```python
from build123d import *

# Parameters (mm, degrees)
EXTRUDE_2_DEPTH     = 3
SKETCH_1_R          = 3.5
CUT_EXTRUDE_2_DEPTH = 4
SKETCH_2_R          = 6.5
CUT_EXTRUDE_4_DEPTH = 2


with BuildPart() as part:
    # Эскиз3 → Бобышка-Вытянуть2 (new body)
    with BuildSketch(Plane(origin=(0, 0, 0), x_dir=(1, 0, 0), z_dir=(0, 1, 0))):
        with BuildLine():
            ThreePointArc((-6.4739783, 66.952525078), (0, 69.5), (6.4739783, 66.952525078))
            ThreePointArc((6.4739783, 66.952525078), (8.677759132, 65.914124613), (11.075205769, 66.34676199))
            ThreePointArc((11.075205769, 66.34676199), (17.987923635, 67.131844927), (23.581971447, 62.995584227))
            ThreePointArc((23.581971447, 62.995584227), (25.441902451, 61.422185949), (27.869632868, 61.219576716))
            ThreePointArc((27.869632868, 61.219576716), (34.75, 60.188765563), (39.082892211, 54.745598415))
            ThreePointArc((39.082892211, 54.745598415), (40.472222163, 52.744426818), (42.764790543, 51.920378458))
            ThreePointArc((42.764790543, 51.920378458), (49.143921292, 49.143921292), (51.920378458, 42.764790543))
            ThreePointArc((51.920378458, 42.764790543), (52.744426818, 40.472222163), (54.745598415, 39.082892211))
            ThreePointArc((54.745598415, 39.082892211), (60.188765563, 34.75), (61.219576716, 27.869632868))
            ThreePointArc((61.219576716, 27.869632868), (61.422185949, 25.441902451), (62.995584227, 23.581971447))
            ThreePointArc((62.995584227, 23.581971447), (67.131844927, 17.987923635), (66.34676199, 11.075205769))
            ThreePointArc((66.34676199, 11.075205769), (65.914124613, 8.677759132), (66.952525078, 6.4739783))
            ThreePointArc((66.952525078, 6.4739783), (69.5, 0), (66.952525078, -6.4739783))
            ThreePointArc((66.952525078, -6.4739783), (65.914124613, -8.677759132), (66.34676199, -11.075205769))
            ThreePointArc((66.34676199, -11.075205769), (67.131844927, -17.987923635), (62.995584227, -23.581971447))
            ThreePointArc((62.995584227, -23.581971447), (61.422185949, -25.441902451), (61.219576716, -27.869632868))
            ThreePointArc((61.219576716, -27.869632868), (60.188765563, -34.75), (54.745598415, -39.082892211))
            ThreePointArc((54.745598415, -39.082892211), (52.744426818, -40.472222163), (51.920378458, -42.764790543))
            ThreePointArc((51.920378458, -42.764790543), (49.143921292, -49.143921292), (42.764790543, -51.920378458))
            ThreePointArc((42.764790543, -51.920378458), (40.472222163, -52.744426818), (39.082892211, -54.745598415))
            ThreePointArc((39.082892211, -54.745598415), (34.75, -60.188765563), (27.869632868, -61.219576716))
            ThreePointArc((27.869632868, -61.219576716), (25.441902451, -61.422185949), (23.581971447, -62.995584227))
            ThreePointArc((23.581971447, -62.995584227), (17.987923635, -67.131844927), (11.075205769, -66.34676199))
            ThreePointArc((11.075205769, -66.34676199), (8.677759132, -65.914124613), (6.4739783, -66.952525078))
            ThreePointArc((6.4739783, -66.952525078), (0, -69.5), (-6.4739783, -66.952525078))
            ThreePointArc((-6.4739783, -66.952525078), (-8.677759132, -65.914124613), (-11.075205769, -66.34676199))
            ThreePointArc((-11.075205769, -66.34676199), (-17.987923635, -67.131844927), (-23.581971447, -62.995584227))
            ThreePointArc((-23.581971447, -62.995584227), (-25.441902451, -61.422185949), (-27.869632868, -61.219576716))
            ThreePointArc((-27.869632868, -61.219576716), (-34.75, -60.188765563), (-39.082892211, -54.745598415))
            ThreePointArc((-39.082892211, -54.745598415), (-40.472222163, -52.744426818), (-42.764790543, -51.920378458))
            ThreePointArc((-42.764790543, -51.920378458), (-49.143921292, -49.143921292), (-51.920378458, -42.764790543))
            ThreePointArc((-51.920378458, -42.764790543), (-52.744426818, -40.472222163), (-54.745598415, -39.082892211))
            ThreePointArc((-54.745598415, -39.082892211), (-60.188765563, -34.75), (-61.219576716, -27.869632868))
            ThreePointArc((-61.219576716, -27.869632868), (-61.422185949, -25.441902451), (-62.995584227, -23.581971447))
            ThreePointArc((-62.995584227, -23.581971447), (-67.131844927, -17.987923635), (-66.34676199, -11.075205769))
            ThreePointArc((-66.34676199, -11.075205769), (-65.914124613, -8.677759132), (-66.952525078, -6.4739783))
            ThreePointArc((-66.952525078, -6.4739783), (-69.5, 0), (-66.952525078, 6.4739783))
            ThreePointArc((-66.952525078, 6.4739783), (-65.914124613, 8.677759132), (-66.34676199, 11.075205769))
            ThreePointArc((-66.34676199, 11.075205769), (-67.131844927, 17.987923635), (-62.995584227, 23.581971447))
            ThreePointArc((-62.995584227, 23.581971447), (-61.422185949, 25.441902451), (-61.219576716, 27.869632868))
            ThreePointArc((-61.219576716, 27.869632868), (-60.188765563, 34.75), (-54.745598415, 39.082892211))
            ThreePointArc((-54.745598415, 39.082892211), (-52.744426818, 40.472222163), (-51.920378458, 42.764790543))
            ThreePointArc((-51.920378458, 42.764790543), (-49.143921292, 49.143921292), (-42.764790543, 51.920378458))
            ThreePointArc((-42.764790543, 51.920378458), (-40.472222163, 52.744426818), (-39.082892211, 54.745598415))
            ThreePointArc((-39.082892211, 54.745598415), (-34.75, 60.188765563), (-27.869632868, 61.219576716))
            ThreePointArc((-27.869632868, 61.219576716), (-25.441902451, 61.422185949), (-23.581971447, 62.995584227))
            ThreePointArc((-23.581971447, 62.995584227), (-17.987923635, 67.131844927), (-11.075205769, 66.34676199))
            ThreePointArc((-11.075205769, 66.34676199), (-8.677759132, 65.914124613), (-6.4739783, 66.952525078))
        make_face()
    extrude(amount=EXTRUDE_2_DEPTH)

    # Эскиз1 → Вырез-Вытянуть2 (cut, through all)
    with BuildSketch(Plane(origin=(0, 0, 0), x_dir=(1, 0, 0), z_dir=(0, 1, 0))):
        with Locations((0, 60)):
            Circle(SKETCH_1_R)
        with Locations((15.529142706, 57.955549577)):
            Circle(SKETCH_1_R)
        with Locations((30, 51.961524227)):
            Circle(SKETCH_1_R)
        with Locations((42.426406871, 42.426406871)):
            Circle(SKETCH_1_R)
        with Locations((51.961524227, 30)):
            Circle(SKETCH_1_R)
        with Locations((57.955549577, 15.529142706)):
            Circle(SKETCH_1_R)
        with Locations((60, 0)):
            Circle(SKETCH_1_R)
        with Locations((57.955549577, -15.529142706)):
            Circle(SKETCH_1_R)
        with Locations((51.961524227, -30)):
            Circle(SKETCH_1_R)
        with Locations((42.426406871, -42.426406871)):
            Circle(SKETCH_1_R)
        with Locations((30, -51.961524227)):
            Circle(SKETCH_1_R)
        with Locations((15.529142706, -57.955549577)):
            Circle(SKETCH_1_R)
        with Locations((0, -60)):
            Circle(SKETCH_1_R)
        with Locations((-15.529142706, -57.955549577)):
            Circle(SKETCH_1_R)
        with Locations((-30, -51.961524227)):
            Circle(SKETCH_1_R)
        with Locations((-42.426406871, -42.426406871)):
            Circle(SKETCH_1_R)
        with Locations((-51.961524227, -30)):
            Circle(SKETCH_1_R)
        with Locations((-57.955549577, -15.529142706)):
            Circle(SKETCH_1_R)
        with Locations((-60, 0)):
            Circle(SKETCH_1_R)
        with Locations((-57.955549577, 15.529142706)):
            Circle(SKETCH_1_R)
        with Locations((-51.961524227, 30)):
            Circle(SKETCH_1_R)
        with Locations((-42.426406871, 42.426406871)):
            Circle(SKETCH_1_R)
        with Locations((-30, 51.961524227)):
            Circle(SKETCH_1_R)
        with Locations((-15.529142706, 57.955549577)):
            Circle(SKETCH_1_R)
    extrude(amount=CUT_EXTRUDE_2_DEPTH, mode=Mode.SUBTRACT)

    # Эскиз2 → Вырез-Вытянуть4 (cut)
    with BuildSketch(Plane(origin=(0, 0, 0), x_dir=(1, 0, 0), z_dir=(0, 1, 0))):
        with Locations((0, 60)):
            Circle(SKETCH_2_R)
        with Locations((15.529142706, 57.955549577)):
            Circle(SKETCH_2_R)
        with Locations((30, 51.961524227)):
            Circle(SKETCH_2_R)
        with Locations((42.426406871, 42.426406871)):
            Circle(SKETCH_2_R)
        with Locations((51.961524227, 30)):
            Circle(SKETCH_2_R)
        with Locations((57.955549577, 15.529142706)):
            Circle(SKETCH_2_R)
        with Locations((60, 0)):
            Circle(SKETCH_2_R)
        with Locations((57.955549577, -15.529142706)):
            Circle(SKETCH_2_R)
        with Locations((51.961524227, -30)):
            Circle(SKETCH_2_R)
        with Locations((42.426406871, -42.426406871)):
            Circle(SKETCH_2_R)
        with Locations((30, -51.961524227)):
            Circle(SKETCH_2_R)
        with Locations((15.529142706, -57.955549577)):
            Circle(SKETCH_2_R)
        with Locations((0, -60)):
            Circle(SKETCH_2_R)
        with Locations((-15.529142706, -57.955549577)):
            Circle(SKETCH_2_R)
        with Locations((-30, -51.961524227)):
            Circle(SKETCH_2_R)
        with Locations((-42.426406871, -42.426406871)):
            Circle(SKETCH_2_R)
        with Locations((-51.961524227, -30)):
            Circle(SKETCH_2_R)
        with Locations((-57.955549577, -15.529142706)):
            Circle(SKETCH_2_R)
        with Locations((-60, 0)):
            Circle(SKETCH_2_R)
        with Locations((-57.955549577, 15.529142706)):
            Circle(SKETCH_2_R)
        with Locations((-51.961524227, 30)):
            Circle(SKETCH_2_R)
        with Locations((-42.426406871, 42.426406871)):
            Circle(SKETCH_2_R)
        with Locations((-30, 51.961524227)):
            Circle(SKETCH_2_R)
        with Locations((-15.529142706, 57.955549577)):
            Circle(SKETCH_2_R)
    extrude(amount=CUT_EXTRUDE_4_DEPTH, mode=Mode.SUBTRACT)


solid = part.part
```
Geometry check sheet. Reference: the model listing, model coordinates, mm. A direction names the side the tool comes from. Give positions to 0.01 mm unless a question says otherwise; leave off trailing zeros. Write each loop counter-clockwise with the first axis right and the second up, starting at its lowest first coordinate (ties: lowest second). Pieces come first, ordered by that corner, then holes. Notation, with made-up numbers: (56.5, -16) -> (60.5, -16) arc R16 cw to (60.5, 2) -> close; hole circle Ø11 at (4, -11). An arc over 180 degrees is marked (long way). Use one line per item in the form item = value.
Item 1: Mould release check, pull along X, two halves, no side actions. Record for faces 3 (the cylindrical face through (-65.92, 1.48, -8.64)), 4 (the cylindrical face through (63.96, 0.99, -13.04)), 5 (the flat face through (-57, 2, 3)): released by +X, released by -X, zero draft, split by the parting line, or undercut.
Results list:
face_3 = released by -X
face_4 = undercut
face_5 = undercut
Item 2: Scan lines: line 1 (X direction, y = 0.6, z = 30); line 2 (Z direction, x = -30, y = 2.55); line 3 (X direction, y = 1.15, z = 15). Record each from-to range of solid material in increasing order.
Results list:
line_1 = -61.46 to -58.46, -45.46 to 45.46, 58.46 to 61.46
line_2 = -61.46 to -55.46, -48.46 to 48.46, 55.46 to 61.46
line_3 = -67.44 to -64.43, -51.48 to 51.48, 64.43 to 67.44
Item 3: Sectioned sample at B-B on z = 30. Enter the section's corners in (x, y), plus the area to 3 significant figures.
Results list:
outline = (-61.46, 0) -> (-58.46, 0) -> (-58.46, 2) -> (-55.46, 2) -> (-55.46, 3) -> (-61.46, 3) -> close; (-48.46, 2) -> (-45.46, 2) -> (-45.46, 0) -> (45.46, 0) -> (45.46, 2) -> (48.46, 2) -> (48.46, 3) -> (-48.46, 3) -> close; (55.46, 2) -> (58.46, 2) -> (58.46, 0) -> (61.46, 0) -> (61.46, 3) -> (55.46, 3) -> close
area = 303 mm2
Item 4: Access from +Z, -Z, +X, -X, +Y, -Y to the whole of each face (thin tool, end or side, straight path). Record for faces 1 (the flat face through (63, 2, 3)), 2 (the cylindrical face through (18.868, 2.493, 56.904)).
Results list:
face_1 = -Y
face_2 = +Y, -Y
Item 5: Sectioned sample at A-A on x = 0. Enter the section's corners in (y, z), plus the area to 3 significant figures.
Results list:
outline = (0, -69.5) -> (3, -69.5) -> (3, -63.5) -> (2, -63.5) -> (2, -66.5) -> (0, -66.5) -> close; (0, -53.5) -> (2, -53.5) -> (2, -56.5) -> (3, -56.5) -> (3, 56.5) -> (2, 56.5) -> (2, 53.5) -> (0, 53.5) -> close; (0, 66.5) -> (2, 66.5) -> (2, 63.5) -> (3, 63.5) -> (3, 69.5) -> (0, 69.5) -> close
area = 351 mm2
Item 6: Sectioned sample at C-C on y = 2.45. Count the separate pieces of the cut face and the enclosed holes in it, plus the area to 3 significant figures.
Results list:
separate_pieces = 1
enclosed_holes = 24
area = 13,700 mm2
Item 7: Depth check by flat-ended pin: pin 1 Ø1 at (x, y) = (-1.5, 1.5) entering from -Z; pin 2 Ø6.5 at (x, z) = (-31, 50.5) entering from -Y; pin 3 Ø1 at (y, z) = (1.5, -36.5) entering from -X; pin 4 Ø5.5 at (x, z) = (-60, 0) entering from -Y. Enter the tip coordinate at first touch or a pass-through.
Results list:
pin_1 = -69.45
pin_2 = 2
pin_3 = -59.33
pin_4 = through
